Job drawing, mm, ordinate dimensions from the low corner. One solid piece. Coordinates: 2 decimals unless noted, no trailing zeros. Loops run counter-clockwise (first coordinate to the right, second up) from the corner with the lowest first, then second, coordinate; pieces in that order, holes last. Notation, with made-up numbers: (12.25, 63.5) - (25.25, 63.5) arc R21 cw to (25.25, 71.5) - close; hole circle Ø2 at (42.5, -29.5). An arc over 180 degrees is marked (long way). Use a Markdown table: item, result. Add a question column.
1. Wall check: probe 1 along Y at (x, z) = (85.5, 2.5) (1 decimal); probe 2 along Y at (x, z) = (85, 5.5); probe 3 along Y at (x, z) = (32.5, 5.5) (1 decimal). Give the ranges that are in metal, low to high. Write a range as [from, to].
2. Band-saw the part on A-A, the plane y = 85.5. Count the separate pieces of the cut face and the enclosed holes in it, plus the area to 3 significant figures.
3. Band-saw the part on C-C, the plane z = 4. Give the cut face in (x, y) (1 decimal).
4. Drop flat-ended pins along their axis: pin 1 (3 mm diameter, centred on x = 146, z = 2.5, fed in from +Y); pin 2 (6 mm diameter, centred on x = 164, y = 85.5, fed in from +Z); pin 3 (1.5 mm diameter, centred on y = 75.5, z = 4, fed in from -X); pin 4 (2 mm diameter, centred on x = 34, z = 3, fed in from +Y). Give the stop position or say it passes through.
5. Band-saw the part on D-D, the plane x = 7. Give the cut face in (y, z), plus the area to 3 significant figures.
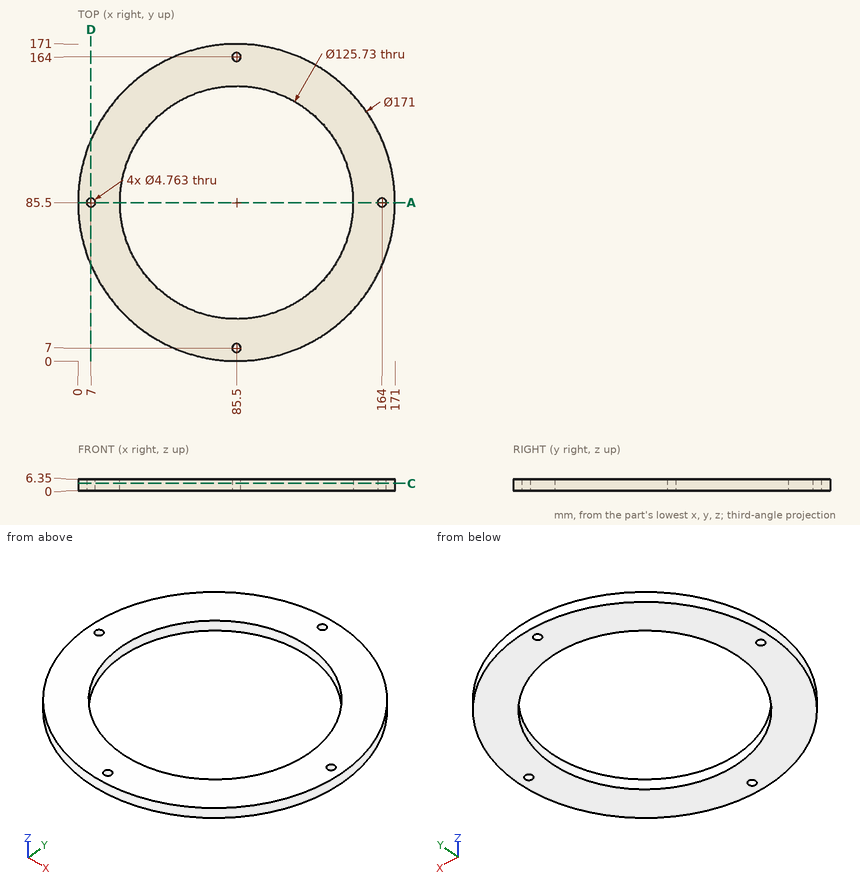
Geometry check:
| question | item | result |
|---|---|---|
| 1 | probe 1 | y = [0, 4.6], [9.4, 22.6], [148.4, 161.6], [166.4, 171] |
| 1 | probe 2 | y = [0, 4.67], [9.33, 22.64], [148.36, 161.67], [166.33, 171] |
| 1 | probe 3 | y = [18.4, 51.7], [119.3, 152.6] |
| 2 | separate pieces | 4 |
| 2 | enclosed holes | 0 |
| 2 | area | 227 mm^2 |
| 3 | outline | circle Ø171 at (85.5, 85.5); hole circle Ø4.8 at (7, 85.5); hole circle Ø125.7 at (85.5, 85.5); hole circle Ø4.8 at (85.5, 7); hole circle Ø4.8 at (85.5, 164); hole circle Ø4.8 at (164, 85.5) |
| 4 | pin 1 | stops at y = 147.38 |
| 4 | pin 2 | stops at z = 6.35 |
| 4 | pin 3 | stops at x = 0.5 |
| 4 | pin 4 | stops at y = 154.49 |
| 5 | outline | (51.62, 0) - (83.12, 0) - (83.12, 6.35) - (51.62, 6.35) - close; (87.88, 0) - (119.38, 0) - (119.38, 6.35) - (87.88, 6.35) - close |
| 5 | area | 400 mm^2 |
